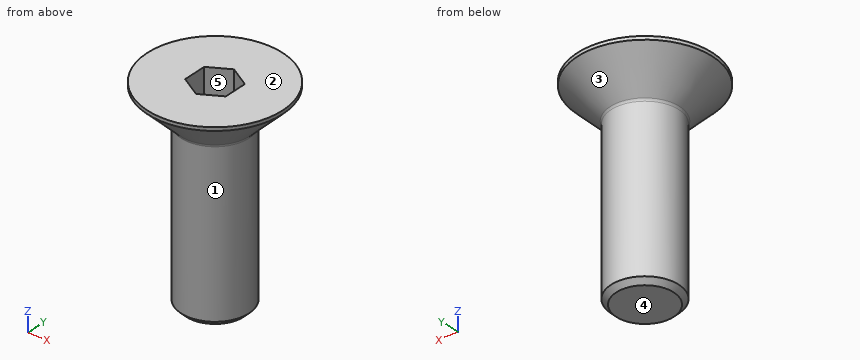
Autodesk Inventor part; units mm, degrees
ref_plane "MSC_PF1" through (0, 0, 0) normal (1, 0, 0) x (0, 1, 0)
ref_plane "MSC_PT1" through (0, 0, 0) normal (0, 0, -1) x (-1, 0, 0)
ref_plane "YZ Plane" through (0, 0, 0) normal (1, 0, 0) x (0, 1, 0)
sketch "Sketch1" plane through (0, 0, 0) normal (0, 1, 0) x (-1, 0, 0)
  point P0 (0, 0)
sketch "Sketch2" plane through (0, 0, 0) normal (0, 1, 0) x (-1, 0, 0)
  line L0 (-5, -30) -> (0, -30)
  line L1 (-5, -5.5) -> (-5, -30)
  line L2 (-10, -0.5) -> (-5, -5.5)
  line L3 (-10, 0) -> (-10, -0.5)
  line L4 (0, 0) -> (-10, 0)
  line L5 (0, -30) -> (0, 0)
  line L6 (0, -30) -> (0, 0)
  line L7 (0, -36) -> (0, 6)
  line L8 (2, 0) -> (-12, 0)
  dimension "d3" = 10
  dimension "d5" = 5
  dimension "d7" = 30
  dimension "ParC" = 0.5
  dimension "d22" = 0
  dimension "d23" = 0
  dimension "d43" = 45
revolve "Revolution1" add sketch "Sketch2" angle 360 about axis through (0, 0, -30) along (0, 0, -1)
sketch "Sketch3" plane through (0, 0, 0) normal (0, 0, 1) x (1, 0, 0)
  line L0 (-3, 1.7321) -> (-3, -1.7321)
  line L1 (0, 3.4641) -> (-3, 1.7321)
  line L2 (3, 1.7321) -> (0, 3.4641)
  line L3 (3, -1.7321) -> (3, 1.7321)
  line L4 (0, -3.4641) -> (3, -1.7321)
  line L5 (-3, -1.7321) -> (0, -3.4641)
  circle A0 centre (0, 0) radius 3 construction
  circle A1 centre (0, 0) radius 5 construction
  dimension "d11" = 6
  dimension "d13" = 120
  dimension "d15" = 120
extrude "Extrusion1" cut sketch "Sketch3" against normal blind 4.4
fillet "Fillet1" radius 0.5 1 edges at (-5, 0, -5.5)
chamfer "Chamfer1" distance 0.75 angle 45 1 edges at (-5, 0, -30) measured on face at (-4.674, 1.7759, -21.9024)
thread "Thread1"
ref_plane "MSC_PF1" through (0, 0, 0) normal (1, 0, 0) x (0, 1, 0)
ref_plane "MSC_PT1" through (0, 0, 0) normal (0, 0, -1) x (-1, 0, 0)
equation "\"d3\" = 0.5 * dk"
equation "\"d5\" = 0.5 * NND"
equation "\"d7\" = NLG"
equation "\"d43\" = 0.5 * ang"
equation "\"d18\" = r"
equation "\"d19\" = 0.5 * PTC"
equation "\"d39\" = 0.5 * PTC"
equation "\"d11\" = ParS"
equation "\"d16\" = ParT"
equation "\"PTC\" = 1.5"
equation "\"ParK\" = 5.5"
equation "\"ParS\" = 6"
equation "\"ParT\" = 4.4"
equation "\"r\" = 0.5"
equation "\"NLG\" = 30"
equation "\"ang\" = 90deg"
properties part number "DIN 7991 - M10x30" material "Steel, Mild"
Build history of the part. All positions in model axes, mm. Face numbers are marked on the shaded views. A direction names the side the tool comes from. Coordinates: 2 decimals unless noted, no trailing zeros. Order: outer loops, then holes, each group sorted by start corner. A loop starts at its lowest first (then second) coordinate and runs counter-clockwise, first axis right, second up. Notation, with made-up numbers: (-5.75, 39) -> (45.25, 39) arc R26 ccw to (45.25, 78) -> close; hole circle Ø8 at (-1.5, -10.5). An arc over 180 degrees is marked (long way). Answer in a Markdown table with one row per item. Add a question column.
Q1. Mould opens along Y. For the marked faces 3, 4 and 5 say: +Y half, -Y half, draft (parallel to the pull), parting line (faces both ways), or undercut.
Q2. Which spindle directions (+Z, -Z, +X, -X, +Y, -Y) get a long thin tool onto all of the face, cutting with end or side? Do the marked faces 1 and 2. Say none if no direction does.
Q3. Band-saw the part on A-A, the plane z = -2.5. List the corners of the cut face in (x, y), then the cut area to 3 significant figures.
Q4. Wall check: line 1 along Y through (x, z) = (4, -20); line 2 along Z through (x, y) = (0, -2.25); line 3 along X through (y, z) = (5.5, -4). Give the ranges that are in metal, low to high. Write a range as [from, to].
Q5. Drop flat-ended pins along their axis: pin 1 (4 mm diameter, centred on y = 0, z = -3.5, fed in from +X); pin 2 (6 mm diameter, centred on x = 0.5, z = -23, fed in from -Y); pin 3 (12 mm diameter, centred on y = -7, z = -3.5, fed in from -X); pin 4 (3 mm diameter, centred on x = 0, y = -7.5, fed in from +Z). Give the stop position or say it passes through.
Q6. Band-saw the part on B-B, the plane z = -19.75. List the corners of the cut face in (x, y), then the cut area to 3 significant figures.
Answers follow:
| question | item | result |
|---|---|---|
| 1 | face 3 | parting line |
| 1 | face 4 | draft |
| 1 | face 5 | undercut |
| 2 | face 1 | -Z |
| 2 | face 2 | +Z, +X, -X, +Y, -Y |
| 3 | outline | circle Ø16 at (0, 0); hole (-3, -1.73) -> (0, -3.46) -> (3, -1.73) -> (3, 1.73) -> (0, 3.46) -> (-3, 1.73) -> close |
| 3 | area | 170 mm^2 |
| 4 | line 1 | [-3, 3] |
| 4 | line 2 | [-30, -4.4] |
| 4 | line 3 | [-3.46, 3.46] |
| 5 | pin 1 | x = 9 |
| 5 | pin 2 | y = -5 |
| 5 | pin 3 | x = -9.84 |
| 5 | pin 4 | z = 0 |
| 6 | outline | circle Ø10 at (0, 0) |
| 6 | area | 78.5 mm^2 |
